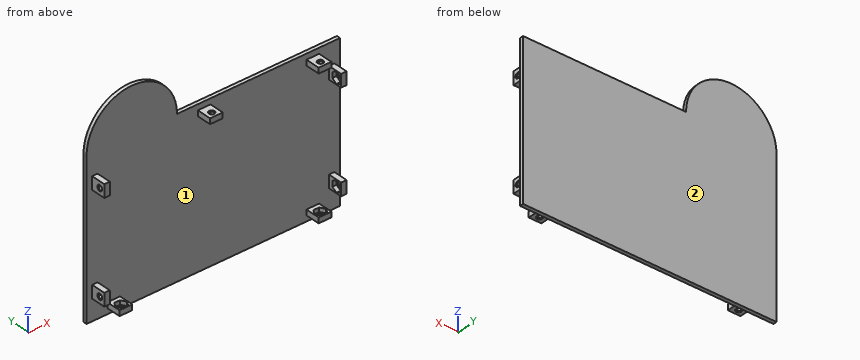
from build123d import *

# Parameters (mm, degrees)
Y_KSEKLIK_EKSTR_ZYON1_DEPTH = 2
IZIM2_W                     = 7
IZIM2_H                     = 3
IZIM2_W_2                   = 3
IZIM2_H_2                   = 7
Y_KSEKLIK_EKSTR_ZYON2_DEPTH = 8
KES_EKSTR_ZYON1_DEPTH       = 2.3
KES_EKSTR_ZYON2_DEPTH       = 2.3
KES_EKSTR_ZYON3_DEPTH       = 2.3
KES_EKSTR_ZYON4_DEPTH       = 2.3
KES_EKSTR_ZYON5_DEPTH       = 2.3
KES_EKSTR_ZYON7_DEPTH       = 2.3
KES_EKSTR_ZYON9_DEPTH       = 2.3
KES_EKSTR_ZYON10_DEPTH      = 2.3
IZIM15_R                    = 1.6
KES_EKSTR_ZYON11_DEPTH      = 5
IZIM16_R                    = 1.6
KES_EKSTR_ZYON12_DEPTH      = 5
IZIM17_R                    = 1.6
KES_EKSTR_ZYON13_DEPTH      = 5
IZIM18_R                    = 1.6
KES_EKSTR_ZYON14_DEPTH      = 5
IZIM19_R                    = 1.6
KES_EKSTR_ZYON15_DEPTH      = 5
KES_EKSTR_ZYON16_START      = -5
IZIM20_R                    = 1.6
KES_EKSTR_ZYON16_DEPTH      = 5
KES_EKSTR_ZYON17_START      = -5
IZIM21_R                    = 1.6
KES_EKSTR_ZYON17_DEPTH      = 5
KES_EKSTR_ZYON18_START      = -5
IZIM22_R                    = 1.6
KES_EKSTR_ZYON18_DEPTH      = 5


with BuildPart() as part:
    # Çizim1 → Yükseklik-Ekstrüzyon1 (new body)
    with BuildSketch(Plane(origin=(0, 0, 0), x_dir=(1, 0, 0), z_dir=(0, 1, 0))):
        with BuildLine():
            Line((50, 0), (140, 0))
            Line((140, 0), (140, 85))
            Line((140, 85), (0, 85))
            Line((0, 85), (0, 0))
            ThreePointArc((0, 0), (25, -25), (50, 0))
        make_face()
    extrude(amount=Y_KSEKLIK_EKSTR_ZYON1_DEPTH)

    # Çizim2 → Yükseklik-Ekstrüzyon2 (add)
    with BuildSketch(Plane.XZ):
        with Locations((15, -80.4)):
            Rectangle(IZIM2_W, IZIM2_H)
        with Locations((125, -80.4)):
            Rectangle(IZIM2_W, IZIM2_H)
        with Locations((4.6, -70)):
            Rectangle(IZIM2_W_2, IZIM2_H_2)
        with Locations((4.6, -15)):
            Rectangle(IZIM2_W_2, IZIM2_H_2)
        with Locations((135.4, -70)):
            Rectangle(IZIM2_W_2, IZIM2_H_2)
        with Locations((135.4, -15)):
            Rectangle(IZIM2_W_2, IZIM2_H_2)
        with Locations((125, -4.6)):
            Rectangle(IZIM2_W, IZIM2_H)
        with Locations((65, -4.6)):
            Rectangle(IZIM2_W, IZIM2_H)
    extrude(amount=Y_KSEKLIK_EKSTR_ZYON2_DEPTH)

    # Çizim3 → Kes-Ekstrüzyon1 (cut)
    with BuildSketch(Plane(origin=(0, 0, -6.1), x_dir=(-1, 0, 0), z_dir=(0, 0, -1))):
        Polygon((-68.175426481, -5), (-66.58771324, -7.75), (-63.41228676, -7.75), (-61.824573519, -5), (-63.41228676, -2.25), (-66.58771324, -2.25), align=None)
    extrude(amount=-KES_EKSTR_ZYON1_DEPTH, mode=Mode.SUBTRACT)

    # Çizim4 → Kes-Ekstrüzyon2 (cut)
    with BuildSketch(Plane(origin=(0, 0, -6.1), x_dir=(-1, 0, 0), z_dir=(0, 0, -1))):
        Polygon((-126.484912109, -2.193156691), (-128.173253665, -4.882549954), (-126.688341556, -7.689393263), (-123.515087891, -7.806843309), (-121.826746335, -5.117450046), (-123.311658444, -2.310606737), align=None)
    extrude(amount=-KES_EKSTR_ZYON2_DEPTH, mode=Mode.SUBTRACT)

    # Çizim5 → Kes-Ekstrüzyon3 (cut)
    with BuildSketch(Plane(origin=(6.1, 0, 0), x_dir=(0, 0, -1), z_dir=(1, 0, 0))):
        Polygon((13.457838364, -2.224199067), (11.825005058, -4.947650687), (13.367166694, -7.72345162), (16.542161636, -7.775800933), (18.174994942, -5.052349313), (16.632833306, -2.27654838), align=None)
    extrude(amount=-KES_EKSTR_ZYON3_DEPTH, mode=Mode.SUBTRACT)

    # Çizim6 → Kes-Ekstrüzyon4 (cut)
    with BuildSketch(Plane(origin=(6.1, 0, 0), x_dir=(0, 0, -1), z_dir=(1, 0, 0))):
        Polygon((68.416764228, -2.247419788), (66.824577724, -4.994832293), (68.407813496, -7.747412505), (71.583235772, -7.752580212), (73.175422276, -5.005167707), (71.592186504, -2.252587495), align=None)
    extrude(amount=-KES_EKSTR_ZYON4_DEPTH, mode=Mode.SUBTRACT)

    # Çizim7 → Kes-Ekstrüzyon5 (cut)
    with BuildSketch(Plane.XY.offset(-78.9)):
        Polygon((13.418242397, -2.246570099), (11.824580957, -4.993127316), (13.40633856, -7.746557217), (16.581757603, -7.753429901), (18.175419043, -5.006872684), (16.59366144, -2.253442783), align=None)
    extrude(amount=-KES_EKSTR_ZYON5_DEPTH, mode=Mode.SUBTRACT)

    # Çizim9 → Kes-Ekstrüzyon7 (cut)
    with BuildSketch(Plane.ZY.offset(-133.9)):
        Polygon((-16.559885261, -2.234120157), (-18.175264838, -4.967960341), (-16.615379578, -7.733840184), (-13.440114739, -7.765879843), (-11.824735162, -5.032039659), (-13.384620422, -2.266159816), align=None)
    extrude(amount=-KES_EKSTR_ZYON7_DEPTH, mode=Mode.SUBTRACT)

    # Çizim11 → Kes-Ekstrüzyon9 (cut)
    with BuildSketch(Plane.ZY.offset(-133.9)):
        Polygon((-71.58771324, -2.25), (-73.175426481, -5), (-71.58771324, -7.75), (-68.41228676, -7.75), (-66.824573519, -5), (-68.41228676, -2.25), align=None)
    extrude(amount=-KES_EKSTR_ZYON9_DEPTH, mode=Mode.SUBTRACT)

    # Çizim12 → Kes-Ekstrüzyon10 (cut)
    with BuildSketch(Plane.XY.offset(-78.9)):
        Polygon((123.41228676, -2.25), (121.824573519, -5), (123.41228676, -7.75), (126.58771324, -7.75), (128.175426481, -5), (126.58771324, -2.25), align=None)
    extrude(amount=-KES_EKSTR_ZYON10_DEPTH, mode=Mode.SUBTRACT)

    # Çizim15 → Kes-Ekstrüzyon11 (cut)
    with BuildSketch(Plane.XY.offset(-3.1)):
        with Locations((125, -5)):
            Circle(IZIM15_R)
    extrude(amount=-KES_EKSTR_ZYON11_DEPTH, mode=Mode.SUBTRACT)

    # Çizim16 → Kes-Ekstrüzyon12 (cut)
    with BuildSketch(Plane.XY.offset(-3.1)):
        with Locations((65, -5)):
            Circle(IZIM16_R)
    extrude(amount=-KES_EKSTR_ZYON12_DEPTH, mode=Mode.SUBTRACT)

    # Çizim17 → Kes-Ekstrüzyon13 (cut)
    with BuildSketch(Plane.ZY.offset(-3.1)):
        with Locations((-15, -5)):
            Circle(IZIM17_R)
    extrude(amount=-KES_EKSTR_ZYON13_DEPTH, mode=Mode.SUBTRACT)

    # Çizim18 → Kes-Ekstrüzyon14 (cut)
    with BuildSketch(Plane.ZY.offset(-3.1)):
        with Locations((-70, -5)):
            Circle(IZIM18_R)
    extrude(amount=-KES_EKSTR_ZYON14_DEPTH, mode=Mode.SUBTRACT)

    # Çizim19 → Kes-Ekstrüzyon15 (cut)
    with BuildSketch(Plane(origin=(0, 0, -81.9), x_dir=(-1, 0, 0), z_dir=(0, 0, -1))):
        with Locations((-15, -5)):
            Circle(IZIM19_R)
    extrude(amount=-KES_EKSTR_ZYON15_DEPTH, mode=Mode.SUBTRACT)

    # Çizim20 → Kes-Ekstrüzyon16 (cut)
    with BuildSketch(Plane(origin=(0, 0, -81.9), x_dir=(-1, 0, 0), z_dir=(0, 0, -1)).offset(KES_EKSTR_ZYON16_START)):
        with Locations(Location((-125, -5, 0), (0, 0, 180))):
            Circle(IZIM20_R)
    extrude(amount=KES_EKSTR_ZYON16_DEPTH, mode=Mode.SUBTRACT)

    # Çizim21 → Kes-Ekstrüzyon17 (cut)
    with BuildSketch(Plane(origin=(136.9, 0, 0), x_dir=(0, 0, -1), z_dir=(1, 0, 0)).offset(KES_EKSTR_ZYON17_START)):
        with Locations(Location((70, -5, 0), (0, 0, 180))):
            Circle(IZIM21_R)
    extrude(amount=KES_EKSTR_ZYON17_DEPTH, mode=Mode.SUBTRACT)

    # Çizim22 → Kes-Ekstrüzyon18 (cut)
    with BuildSketch(Plane(origin=(136.9, 0, 0), x_dir=(0, 0, -1), z_dir=(1, 0, 0)).offset(KES_EKSTR_ZYON18_START)):
        with Locations(Location((15, -5, 0), (0, 0, 180))):
            Circle(IZIM22_R)
    extrude(amount=KES_EKSTR_ZYON18_DEPTH, mode=Mode.SUBTRACT)


solid = part.part
Design review of the part built by this model. Coordinates are the model's own, in mm. Face numbers are marked on the shaded views. Coordinates: 2 decimals unless noted, no trailing zeros. Write each loop counter-clockwise with the first axis right and the second up, starting at its lowest first coordinate (ties: lowest second). Pieces come first, ordered by that corner, then holes. Notation, with made-up numbers: (12.25, -4) -> (50.25, -4) arc R9 ccw to (50.25, 12) -> close; hole circle Ø2 at (64.25, 34). An arc over 180 degrees is marked (long way). Write each question's results on one line, items separated by ' | '. Start each with the question number.
(1) Take a section at A-A on z = -70. Write out the cut boundary in (x, y).
(2) Take a section at C-C on z = -47. Write out the cut boundary in (x, y).
(3) For line 1 along Y through (x, z) = (136.65, -15); line 2 along Z through (x, y) = (122, -5.25); line 3 along Y through (x, z) = (125, -3), list the stretches that pass through material, from the lowest coordinate up. Write a range as from..to.
(4) Clearance check with flat-ended pins moving along their axes: P1, Ø2, axis at y = -2.5, z = -15.5, coming from the +X side; P2, Ø2, axis at y = -3.5, z = -72.5, coming from the -X side; P3, Ø2, axis at x = 124, y = -3, coming from the -Z side; P4, Ø2.5, axis at y = -5, z = -70, coming from the -X side. State where each tip first meets the part, or that it passes through.
(5) Take a section at B-B on x = 15. Write out the cut boundary in (y, z), and give its area (3 significant figures).
(6) Take a section at D-D on x = 71. Write out the cut boundary in (y, z).
(7) The part is to be moulded in two halves that separate along X. For the marked faces 1 and 2, say which applies: pulls with the +X half, pulls with the -X half, needs draft (parallel to the pull), parting line crosses it, or undercut.
Results found:
1) outline: (0, 0) -> (3.1, 0) -> (3.1, -3.4) -> (3.8, -3.4) -> (3.8, -2.25) -> (6.1, -2.25) -> (6.1, 0) -> (133.9, 0) -> (133.9, -2.25) -> (136.2, -2.25) -> (136.2, -3.4) -> (136.9, -3.4) -> (136.9, 0) -> (140, 0) -> (140, 2) -> (0, 2) -> close; (3.1, -8) -> (6.1, -8) -> (6.1, -7.75) -> (3.8, -7.75) -> (3.8, -6.6) -> (3.1, -6.6) -> close; (133.9, -8) -> (136.9, -8) -> (136.9, -6.6) -> (136.2, -6.6) -> (136.2, -7.75) -> (133.9, -7.75) -> close
2) outline: (0, 0) -> (140, 0) -> (140, 2) -> (0, 2) -> close
3) line 1: y = -8..-6.6, -3.4..2 | line 2: z = -81.9..-81.2, -3.8..-3.1 | line 3: y = 0..2
4) P1: stops at x = 136.9 | P2: stops at x = 3.1 | P3: stops at z = -81.9 | P4: passes through
5) outline: (-8, -81.9) -> (-6.6, -81.9) -> (-6.6, -81.2) -> (-7.75, -81.2) -> (-7.75, -78.9) -> (-8, -78.9) -> close; (-3.4, -81.9) -> (0, -81.9) -> (0, -85) -> (2, -85) -> (2, 22.91) -> (0, 22.91) -> (0, -78.9) -> (-2.25, -78.9) -> (-2.25, -81.2) -> (-3.4, -81.2) -> close | area: 225 mm2
6) outline: (0, -85) -> (2, -85) -> (2, 0) -> (0, 0) -> close
7) face 1: undercut | face 2: needs draft
